Could you check a few things on this model? Use its own coordinates, in mm. Give positions to 0.01 mm unless a question says otherwise; leave off trailing zeros. Loops run counter-clockwise (first coordinate to the right, second up) from the corner with the lowest first, then second, coordinate; pieces in that order, holes last.
1. For P1, Ø1.5, axis at x = -57, z = 3.5, coming from the -Y side; P2, Ø1.5, axis at x = 58.5, z = 1.5, coming from the +Y side; P3, Ø1, axis at y = 23, z = 2, coming from the +X side; P4, Ø10, axis at x = -47.5, y = -16, coming from the +Z side, each with a flat end and sliding along its axis, tell me the tip position at first contact or that it passes through.
2. I need wall thicknesses on line 1 along X through (y, z) = (1.5, 2.45); line 2 along Y through (x, z) = (0, 2.7); line 3 along X through (y, z) = (-31, 0.55). Which ranges of each line are inside material? Lowest first, please.
3. Imagine slicing it at D-D (x = 52). List the corners of the cut face in (y, z) for me, plus the area to 3 significant figures.
4. Imagine slicing it at A-A (y = 0). List the corners of the cut face in (x, z) for me.
5. Imagine slicing it at B-B (x = 0). List the corners of the cut face in (y, z) for me, plus the area to 3 significant figures.
6. Imagine slicing it at C-C (y = -19). List the corners of the cut face in (x, z) for me, plus the area to 3 significant figures.
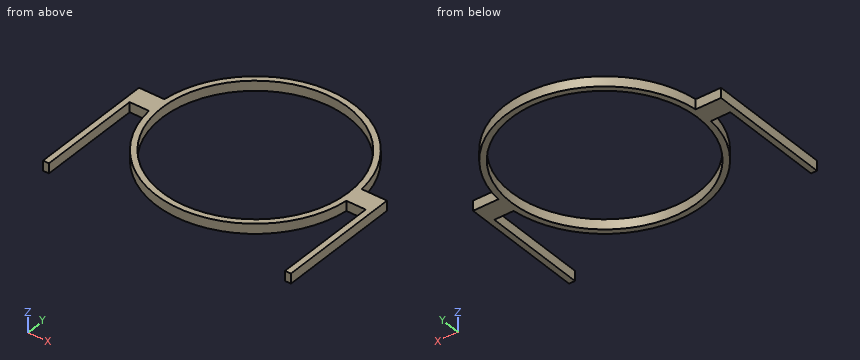
Autodesk Inventor part; units mm, degrees
ref_plane "YZ Plane" through (0, 0, 0) normal (1, 0, 0) x (0, 1, 0)
ref_plane "XZ Plane" through (0, 0, 0) normal (0, 1, 0) x (-1, 0, 0)
ref_plane "XY Plane" through (0, 0, 0) normal (0, 0, 1) x (1, 0, 0)
sketch "Sketch1" plane through (0, 0, 0) normal (0, 0, 1) x (1, 0, 0)
  circle A0 centre (0, 0) radius 50
  circle A1 centre (0, 0) radius 47
  line L0 (37.5, 5) -> (62.5, 5)
  line L1 (62.5, 5) -> (62.5, -5)
  line L2 (62.5, -5) -> (37.5, -5)
  line L3 (37.5, -5) -> (37.5, 5)
  line L4 (37.5, 5) -> (62.5, -5) construction
  line L5 (62.5, 5) -> (37.5, -5) construction
  line L6 (-62.5, 5) -> (-37.5, 5)
  line L7 (-37.5, 5) -> (-37.5, -5)
  line L8 (-37.5, -5) -> (-62.5, -5)
  line L9 (-62.5, -5) -> (-62.5, 5)
  line L10 (-62.5, 5) -> (-37.5, -5) construction
  line L11 (-37.5, 5) -> (-62.5, -5) construction
  line L12 (62.5, 0) -> (59.5, 0)
  line L13 (59.5, 0) -> (59.5, -57.5)
  line L14 (59.5, -57.5) -> (62.5, -57.5)
  line L15 (62.5, -57.5) -> (62.5, 0)
  line L16 (-62.5, 0) -> (-59.5, 0)
  line L17 (-59.5, 0) -> (-59.5, -57.5)
  line L18 (-59.5, -57.5) -> (-62.5, -57.5)
  line L19 (-62.5, -57.5) -> (-62.5, 0)
  point P0 (50, 0)
  point P1 (-50, 0)
  point P2 (49.7494, 5)
  point P3 (-49.7494, 5)
  point P4 (-59.5, -5)
  point P5 (-49.7494, -5)
  point P6 (49.7494, -5)
  point P7 (59.5, -5)
  dimension "d0" = 100
  dimension "d1" = 94
  dimension "d2" = 25
  dimension "d3" = 10
  dimension "d4" = 25
  dimension "d5" = 10
  dimension "d6" = 3
  dimension "d7" = 57.5
  dimension "d8" = 3
  dimension "d9" = 57.5
extrude "Extrusion1" add sketch "Sketch1" along normal blind 5 contours A0 L2 A1 L0 | A0 L0 L1 L12 L13 L2 | L0 A1 L6 A0 | A0 L8 A1 L2 | L6 A1 L8 A0 | A0 L8 L17 L16 L9 L6 | L13 L12 L1 L2 | L2 L15 L14 L13 | L17 L18 L19 L8 | L8 L9 L16 L17
properties part number "PIEZA_JACLUBER_2" material "Steel, Mild, Welded"
Derived:
1. P1: stops at y = -5
1. P2: stops at y = 5
1. P3: stops at x = 44.65
1. P4: stops at z = 5
2. line 1: x = -62.5 to -46.98, 46.98 to 62.5
2. line 2: y = -50 to -47, 47 to 50
2. line 3: x = -62.5 to -59.5, -39.23 to -35.33, 35.33 to 39.23, 59.5 to 62.5
3. outline: (-5, 0) - (5, 0) - (5, 5) - (-5, 5) - close
3. area: 50.0 mm2
4. outline: (-62.5, 0) - (-47, 0) - (-47, 5) - (-62.5, 5) - close; (47, 0) - (62.5, 0) - (62.5, 5) - (47, 5) - close
5. outline: (-50, 0) - (-47, 0) - (-47, 5) - (-50, 5) - close; (47, 0) - (50, 0) - (50, 5) - (47, 5) - close
5. area: 30.0 mm2
6. outline: (-62.5, 0) - (-59.5, 0) - (-59.5, 5) - (-62.5, 5) - close; (-46.25, 0) - (-42.99, 0) - (-42.99, 5) - (-46.25, 5) - close; (42.99, 0) - (46.25, 0) - (46.25, 5) - (42.99, 5) - close; (59.5, 0) - (62.5, 0) - (62.5, 5) - (59.5, 5) - close
6. area: 62.6 mm2
